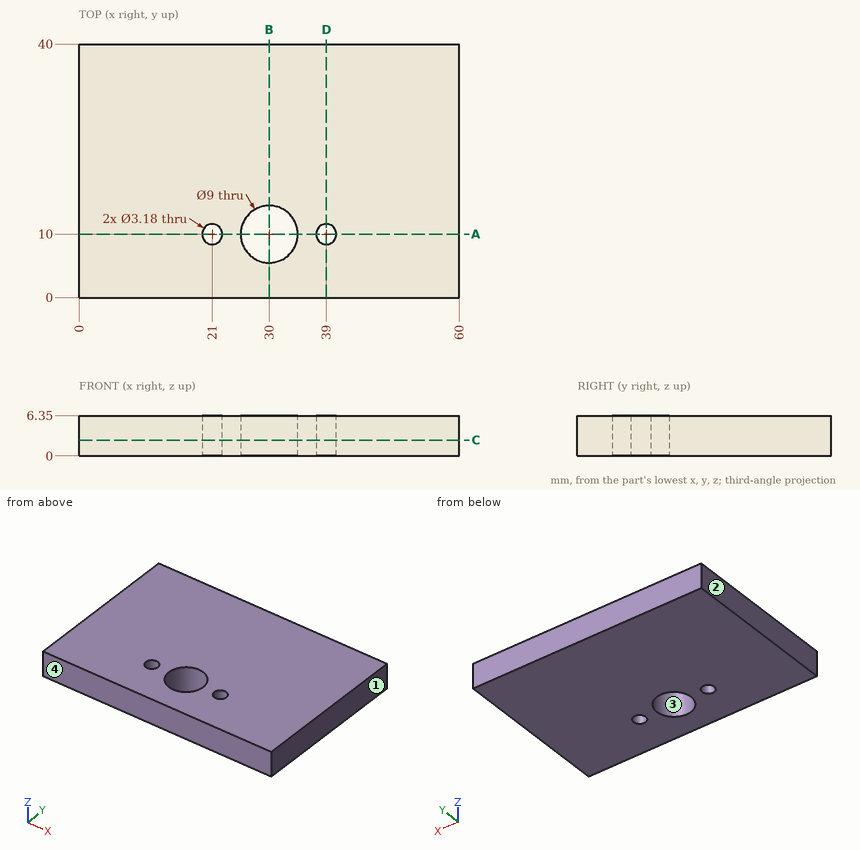
Design review of the part shown in the three views and the two pictorial views. Dimensions are in mm from the part's minimum x, y and z. Give positions to 0.01 mm unless a question says otherwise; leave off trailing zeros. Write each loop counter-clockwise with the first axis right and the second up, starting at its lowest first coordinate (ties: lowest second). Pieces come first, ordered by that corner, then holes. Notation, with made-up numbers: (77.5, -3) -> (134.5, -3) arc R14 ccw to (134.5, 4) -> close; hole circle Ø7 at (3, -30.75). An arc over 180 degrees is marked (long way). Answer in a Markdown table with one row per item.
1) Add section B-B on x = 30. State the section outline as (y, z) points, plus the area to 3 significant figures.
Worked answers:
| item | result |
|---|---|
| outline | (0, 0) -> (5.5, 0) -> (5.5, 6.35) -> (0, 6.35) -> close; (14.5, 0) -> (40, 0) -> (40, 6.35) -> (14.5, 6.35) -> close |
| area | 197 mm² |
2) Add section A-A on y = 10. State the section outline as (x, z) points.
Worked answers:
| item | result |
|---|---|
| outline | (0, 0) -> (19.41, 0) -> (19.41, 6.35) -> (0, 6.35) -> close; (22.59, 0) -> (25.5, 0) -> (25.5, 6.35) -> (22.59, 6.35) -> close; (34.5, 0) -> (37.41, 0) -> (37.41, 6.35) -> (34.5, 6.35) -> close; (40.59, 0) -> (60, 0) -> (60, 6.35) -> (40.59, 6.35) -> close |
3) Add section C-C on z = 2.5. State the section outline as (x, y) points.
Worked answers:
| item | result |
|---|---|
| outline | (0, 0) -> (60, 0) -> (60, 40) -> (0, 40) -> close; hole circle Ø3.18 at (21, 10); hole circle Ø9 at (30, 10); hole circle Ø3.18 at (39, 10) |
4) Add section D-D on x = 39. State the section outline as (y, z) points.
Worked answers:
| item | result |
|---|---|
| outline | (0, 0) -> (8.41, 0) -> (8.41, 6.35) -> (0, 6.35) -> close; (11.59, 0) -> (40, 0) -> (40, 6.35) -> (11.59, 6.35) -> close |
5) Mouldability with a two-part tool opening along X and no side actions: class the marked faces 1, 2, 3 and 4 as +X half, -X half, draft (parallel to the pull), parting line (faces both ways), or undercut.
Worked answers:
| item | result |
|---|---|
| face 1 | +X half |
| face 2 | -X half |
| face 3 | undercut |
| face 4 | draft |
6) For L1, parallel to Y at x = 30, z = 2.5; L2, parallel to Y at x = 39, z = 4.25; L3, parallel to X at y = 7.5, z = 3.5, list the stretches that pass through material, from the lowest coordinate up. Write a range as [from, to].
Worked answers:
| item | result |
|---|---|
| L1 | [0, 5.5], [14.5, 40] |
| L2 | [0, 8.41], [11.59, 40] |
| L3 | [0, 26.26], [33.74, 60] |
